from build123d import *

# Parameters (mm, degrees)
F1_DEPTH = 0.9
F2_DEPTH = 0.5
F3_DEPTH = 1.3


with BuildPart() as f1:
    # F0 (on Front) → F1 (new body)
    with BuildSketch(Plane.XZ):
        with BuildLine():
            ThreePointArc((0, 20), (5.857864, 5.857864), (20, 0))
            Line((20, 0), (65, 0))
            Line((65, 0), (110, 0))
            ThreePointArc((110, 0), (124.142136, 5.857864), (130, 20))
            Line((130, 20), (130, 110))
            ThreePointArc((130, 110), (124.142136, 124.142136), (110, 130))
            Line((110, 130), (65, 130))
            Line((65, 130), (20, 130))
            ThreePointArc((20, 130), (5.857864, 124.142136), (0, 110))
            Line((0, 110), (0, 20))
        make_face()
        with BuildLine():
            Line((65, 120), (110, 120))
            ThreePointArc((110, 120), (117.071068, 117.071068), (120, 110))
            Line((120, 110), (120, 20))
            ThreePointArc((120, 20), (117.071068, 12.928932), (110, 10))
            Line((110, 10), (65, 10))
            Line((65, 10), (20, 10))
            ThreePointArc((20, 10), (12.928932, 12.928932), (10, 20))
            Line((10, 20), (10, 110))
            ThreePointArc((10, 110), (12.928932, 117.071068), (20, 120))
            Line((20, 120), (65, 120))
        make_face(mode=Mode.SUBTRACT)
        with BuildLine():
            ThreePointArc((120, 110), (117.071068, 117.071068), (110, 120))
            Line((110, 120), (65, 120))
            Line((65, 120), (20, 120))
            ThreePointArc((20, 120), (12.928932, 117.071068), (10, 110))
            Line((10, 110), (10, 20))
            ThreePointArc((10, 20), (12.928932, 12.928932), (20, 10))
            Line((20, 10), (65, 10))
            Line((65, 10), (110, 10))
            ThreePointArc((110, 10), (117.071068, 12.928932), (120, 20))
            Line((120, 20), (120, 110))
        make_face()
        with BuildLine():
            ThreePointArc((50.480648, 88.216089), (54.456949, 93.842425), (61, 96))
            Line((61, 96), (65, 96))
            Line((65, 96), (69, 96))
            ThreePointArc((69, 96), (75.543051, 93.842425), (79.519352, 88.216089))
            Line((79.519352, 88.216089), (86.390087, 65.742927))
            ThreePointArc((86.390087, 65.742927), (84.398288, 61.996898), (80.652259, 63.988697))
            Line((80.652259, 63.988697), (75.828126, 79.767725))
            ThreePointArc((75.828126, 79.767725), (74.847274, 80.30417), (74.287869, 79.336229))
            Line((74.287869, 79.336229), (81.450841, 51.234772))
            ThreePointArc((81.450841, 51.234772), (81.002351, 49.083284), (79.028301, 48.117275))
            Line((79.028301, 48.117275), (74.628301, 48.117275))
            ThreePointArc((74.628301, 48.117275), (73.214088, 47.531488), (72.628301, 46.117275))
            Line((72.628301, 46.117275), (72.628301, 21.117275))
            ThreePointArc((72.628301, 21.117275), (69.128301, 17.617275), (65.628301, 21.117275))
            Line((65.628301, 21.117275), (65.628301, 45.488974))
            ThreePointArc((65.628301, 45.488974), (65.444276, 45.93325), (65, 46.117275))
            ThreePointArc((65, 46.117275), (64.555724, 45.93325), (64.371699, 45.488974))
            Line((64.371699, 45.488974), (64.371699, 21.117275))
            ThreePointArc((64.371699, 21.117275), (60.871699, 17.617275), (57.371699, 21.117275))
            Line((57.371699, 21.117275), (57.371699, 46.117275))
            ThreePointArc((57.371699, 46.117275), (56.785912, 47.531488), (55.371699, 48.117275))
            Line((55.371699, 48.117275), (50.971699, 48.117275))
            ThreePointArc((50.971699, 48.117275), (48.997649, 49.083284), (48.549159, 51.234772))
            Line((48.549159, 51.234772), (55.712131, 79.336229))
            ThreePointArc((55.712131, 79.336229), (55.152726, 80.30417), (54.171874, 79.767725))
            Line((54.171874, 79.767725), (49.347741, 63.988697))
            ThreePointArc((49.347741, 63.988697), (45.601712, 61.996898), (43.609913, 65.742927))
            Line((43.609913, 65.742927), (50.480648, 88.216089))
        make_face(mode=Mode.SUBTRACT)
        with BuildLine():
            ThreePointArc((65, 98.5), (57.5, 106), (65, 113.5))
            ThreePointArc((65, 113.5), (72.5, 106), (65, 98.5))
        make_face(mode=Mode.SUBTRACT)
        with BuildLine():
            Line((65, 96), (61, 96))
            ThreePointArc((61, 96), (54.456949, 93.842425), (50.480648, 88.216089))
            Line((50.480648, 88.216089), (43.609913, 65.742927))
            ThreePointArc((43.609913, 65.742927), (45.601712, 61.996898), (49.347741, 63.988697))
            Line((49.347741, 63.988697), (54.171874, 79.767725))
            ThreePointArc((54.171874, 79.767725), (55.152726, 80.30417), (55.712131, 79.336229))
            Line((55.712131, 79.336229), (48.549159, 51.234772))
            ThreePointArc((48.549159, 51.234772), (48.997649, 49.083284), (50.971699, 48.117275))
            Line((50.971699, 48.117275), (55.371699, 48.117275))
            ThreePointArc((55.371699, 48.117275), (56.785912, 47.531488), (57.371699, 46.117275))
            Line((57.371699, 46.117275), (57.371699, 21.117275))
            ThreePointArc((57.371699, 21.117275), (60.871699, 17.617275), (64.371699, 21.117275))
            Line((64.371699, 21.117275), (64.371699, 45.488974))
            ThreePointArc((64.371699, 45.488974), (64.555724, 45.93325), (65, 46.117275))
            ThreePointArc((65, 46.117275), (65.444276, 45.93325), (65.628301, 45.488974))
            Line((65.628301, 45.488974), (65.628301, 21.117275))
            ThreePointArc((65.628301, 21.117275), (69.128301, 17.617275), (72.628301, 21.117275))
            Line((72.628301, 21.117275), (72.628301, 46.117275))
            ThreePointArc((72.628301, 46.117275), (73.214088, 47.531488), (74.628301, 48.117275))
            Line((74.628301, 48.117275), (79.028301, 48.117275))
            ThreePointArc((79.028301, 48.117275), (81.002351, 49.083284), (81.450841, 51.234772))
            Line((81.450841, 51.234772), (74.287869, 79.336229))
            ThreePointArc((74.287869, 79.336229), (74.847274, 80.30417), (75.828126, 79.767725))
            Line((75.828126, 79.767725), (80.652259, 63.988697))
            ThreePointArc((80.652259, 63.988697), (84.398288, 61.996898), (86.390087, 65.742927))
            Line((86.390087, 65.742927), (79.519352, 88.216089))
            ThreePointArc((79.519352, 88.216089), (75.543051, 93.842425), (69, 96))
            Line((69, 96), (65, 96))
        make_face()
        with BuildLine():
            ThreePointArc((65, 98.5), (72.5, 106), (65, 113.5))
            ThreePointArc((65, 113.5), (57.5, 106), (65, 98.5))
        make_face()
    extrude(amount=-F1_DEPTH)

    # F0 (on Front) → F2 (join)
    with BuildSketch(Plane.XZ):
        with BuildLine():
            ThreePointArc((0, 20), (5.857864, 5.857864), (20, 0))
            Line((20, 0), (65, 0))
            Line((65, 0), (110, 0))
            ThreePointArc((110, 0), (124.142136, 5.857864), (130, 20))
            Line((130, 20), (130, 110))
            ThreePointArc((130, 110), (124.142136, 124.142136), (110, 130))
            Line((110, 130), (65, 130))
            Line((65, 130), (20, 130))
            ThreePointArc((20, 130), (5.857864, 124.142136), (0, 110))
            Line((0, 110), (0, 20))
        make_face()
        with BuildLine():
            Line((65, 120), (110, 120))
            ThreePointArc((110, 120), (117.071068, 117.071068), (120, 110))
            Line((120, 110), (120, 20))
            ThreePointArc((120, 20), (117.071068, 12.928932), (110, 10))
            Line((110, 10), (65, 10))
            Line((65, 10), (20, 10))
            ThreePointArc((20, 10), (12.928932, 12.928932), (10, 20))
            Line((10, 20), (10, 110))
            ThreePointArc((10, 110), (12.928932, 117.071068), (20, 120))
            Line((20, 120), (65, 120))
        make_face(mode=Mode.SUBTRACT)
    extrude(amount=F2_DEPTH)

    # F0 (on Front) → F3 (join)
    with BuildSketch(Plane.XZ):
        with BuildLine():
            ThreePointArc((65, 98.5), (72.5, 106), (65, 113.5))
            ThreePointArc((65, 113.5), (57.5, 106), (65, 98.5))
        make_face()
        with BuildLine():
            Line((65, 96), (61, 96))
            ThreePointArc((61, 96), (54.456949, 93.842425), (50.480648, 88.216089))
            Line((50.480648, 88.216089), (43.609913, 65.742927))
            ThreePointArc((43.609913, 65.742927), (45.601712, 61.996898), (49.347741, 63.988697))
            Line((49.347741, 63.988697), (54.171874, 79.767725))
            ThreePointArc((54.171874, 79.767725), (55.152726, 80.30417), (55.712131, 79.336229))
            Line((55.712131, 79.336229), (48.549159, 51.234772))
            ThreePointArc((48.549159, 51.234772), (48.997649, 49.083284), (50.971699, 48.117275))
            Line((50.971699, 48.117275), (55.371699, 48.117275))
            ThreePointArc((55.371699, 48.117275), (56.785912, 47.531488), (57.371699, 46.117275))
            Line((57.371699, 46.117275), (57.371699, 21.117275))
            ThreePointArc((57.371699, 21.117275), (60.871699, 17.617275), (64.371699, 21.117275))
            Line((64.371699, 21.117275), (64.371699, 45.488974))
            ThreePointArc((64.371699, 45.488974), (64.555724, 45.93325), (65, 46.117275))
            ThreePointArc((65, 46.117275), (65.444276, 45.93325), (65.628301, 45.488974))
            Line((65.628301, 45.488974), (65.628301, 21.117275))
            ThreePointArc((65.628301, 21.117275), (69.128301, 17.617275), (72.628301, 21.117275))
            Line((72.628301, 21.117275), (72.628301, 46.117275))
            ThreePointArc((72.628301, 46.117275), (73.214088, 47.531488), (74.628301, 48.117275))
            Line((74.628301, 48.117275), (79.028301, 48.117275))
            ThreePointArc((79.028301, 48.117275), (81.002351, 49.083284), (81.450841, 51.234772))
            Line((81.450841, 51.234772), (74.287869, 79.336229))
            ThreePointArc((74.287869, 79.336229), (74.847274, 80.30417), (75.828126, 79.767725))
            Line((75.828126, 79.767725), (80.652259, 63.988697))
            ThreePointArc((80.652259, 63.988697), (84.398288, 61.996898), (86.390087, 65.742927))
            Line((86.390087, 65.742927), (79.519352, 88.216089))
            ThreePointArc((79.519352, 88.216089), (75.543051, 93.842425), (69, 96))
            Line((69, 96), (65, 96))
        make_face()
    extrude(amount=F3_DEPTH)


solid = f1.part
The listing builds one solid part. Answer for the finished solid, in the listing's coordinates (mm). A direction names the side the tool comes from. Give positions to 0.01 mm unless a question says otherwise; leave off trailing zeros. Write each loop counter-clockwise with the first axis right and the second up, starting at its lowest first coordinate (ties: lowest second). Pieces come first, ordered by that corner, then holes.
1) Find the intervals of material crossed by L1, parallel to X at y = -0.05, z = 105.5; L2, parallel to X at y = -0.45, z = 97, in increasing order.
2) A tool of negligible diameter and unlimited length cuts with its end or side. For faces 5 (the face through (5.703, 0.21, 6.014)), 6 (the face through (83.003, -0.641, 76.822)), from which of +Z, -Z, +X, -X, +Y, -Y can it reach the whole face along a straight path? Write none if from no direction.
3) Section B-B (x = 41) is taken. Write down the section's boundary in (y, z).
4) Section D-D (z = 85) is taken. Write down the section's boundary in (x, y), and give its area (3 significant figures).
5) Given P1, Ø0.6, axis at x = 76, y = -1, coming from the -Z side; P2, Ø2, axis at x = 43.5, z = 103, coming from the -Y side, each flat-ended and moving along its own axis, determine where each tip first touches the part or whether it passes through.
6) Section C-C (z = 106) is taken. Write down the section's boundary in (x, y), and give its area (4 significant figures).
7) Section A-A (y = -0.9) is taken. Write down the section's boundary in (x, z), and give its area (3 significant figures).
8) For a pull along X with two mould halves and no side action, classify faces 1 (the face through (123.986, 0.21, 5.703)), 2 (the face through (51.726, -0.641, 71.768)), 3 (the face through (65, -1.3, 106)), 4 (the face through (6.014, 0.21, 124.297)) as pulls with the +X half, pulls with the -X half, needs draft (parallel to the pull), parting line crosses it, or undercut.
Response:
1. L1: x = 0 to 10, 57.52 to 72.48, 120 to 130
1. L2: x = 0 to 10, 120 to 130
2. face 5: -Z, -X, +Y, -Y
2. face 6: -Y
3. outline: (-0.5, 0) - (0.9, 0) - (0.9, 130) - (-0.5, 130) - (-0.5, 120) - (0, 120) - (0, 10) - (-0.5, 10) - close
4. outline: (0, -0.5) - (10, -0.5) - (10, 0) - (49.5, 0) - (49.5, -1.3) - (80.5, -1.3) - (80.5, 0) - (120, 0) - (120, -0.5) - (130, -0.5) - (130, 0.9) - (0, 0.9) - close
4. area: 167 mm2
5. P1: stops at z = 48.12
5. P2: stops at y = 0
6. outline: (0, -0.5) - (10, -0.5) - (10, 0) - (57.5, 0) - (57.5, -1.3) - (72.5, -1.3) - (72.5, 0) - (120, 0) - (120, -0.5) - (130, -0.5) - (130, 0.9) - (0, 0.9) - close
6. area: 146.5 mm2
7. outline: (43.61, 65.74) arc R3 ccw to (49.35, 63.99) - (54.17, 79.77) arc R0.8 cw to (55.71, 79.34) - (48.55, 51.23) arc R2.5 ccw to (50.97, 48.12) - (55.37, 48.12) arc R2 cw to (57.37, 46.12) - (57.37, 21.12) arc R3.5 ccw to (64.37, 21.12) - (64.37, 45.49) arc R0.63 cw to (65.63, 45.49) - (65.63, 21.12) arc R3.5 ccw to (72.63, 21.12) - (72.63, 46.12) arc R2 cw to (74.63, 48.12) - (79.03, 48.12) arc R2.5 ccw to (81.45, 51.23) - (74.29, 79.34) arc R0.8 cw to (75.83, 79.77) - (80.65, 63.99) arc R3 ccw to (86.39, 65.74) - (79.52, 88.22) arc R11 ccw to (69, 96) - (61, 96) arc R11 ccw to (50.48, 88.22) - close; circle Ø15 at (65, 106)
7. area: 2,090 mm2
8. face 1: pulls with the +X half
8. face 2: undercut
8. face 3: needs draft
8. face 4: pulls with the -X half
